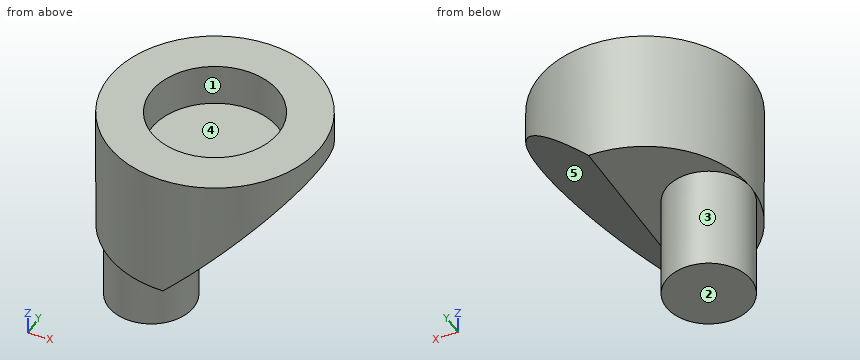
```python
from build123d import *

# Parameters (mm, degrees)
F0_R          = 2.5
F1_DEPTH      = 3
F3_DEPTH      = 25
F3_DEPTH_BACK = 25
F4_R          = 1
F5_DEPTH      = 2.5
F6_R          = 1.5
F7_DEPTH      = 1


with BuildPart() as f1:
    # F0 (on Top) → F1 (new body)
    with BuildSketch(Plane.XY):
        Circle(F0_R)
    extrude(amount=F1_DEPTH)

    # F2 (on Front) → F3 (cut, two sides)
    with BuildSketch(Plane.XZ) as f3_sk:
        Polygon((6.7282968301, 6.6747666272), (-4.7879227272, -4.8414529301), (6.7282968301, -4.8414529301), align=None)
    extrude(amount=-F3_DEPTH, mode=Mode.SUBTRACT)
    extrude(f3_sk.sketch, amount=F3_DEPTH_BACK, mode=Mode.SUBTRACT)

    # F4 (on face) → F5 (join)
    with BuildSketch(Plane(origin=(0, 0, 0), x_dir=(1, 0, 0), z_dir=(0, 0, -1))):
        with Locations((-1.5, 0)):
            Circle(F4_R)
    extrude(amount=F5_DEPTH)

    # F6 (on face) → F7 (cut)
    with BuildSketch(Plane.XY.offset(3)):
        Circle(F6_R)
    extrude(amount=-F7_DEPTH, mode=Mode.SUBTRACT)


solid = f1.part
```
Geometry: final body of the model. Coordinates: model frame, mm. Face numbers are marked on the shaded views. A direction names the side the tool comes from. Give positions to 0.01 mm unless a question says otherwise; leave off trailing zeros. Loops run counter-clockwise (first coordinate to the right, second up) from the corner with the lowest first, then second, coordinate; pieces in that order, holes last. Notation, with made-up numbers: (8, 54.25) -> (35, 54.25) arc R21 ccw to (35, 77.25) -> close; hole circle Ø2 at (23.25, 17.25). An arc over 180 degrees is marked (long way). Use CSV: the item, a comma, the result in double quotes.
(1) Cut plane B-B (x = -0.8). Output: boundary loops of the cut face in (y, z).
From the geometry:
outline,"(-2.37, 0) -> (-0.71, 0) -> (-0.71, -2.5) -> (0.71, -2.5) -> (0.71, 0) -> (2.37, 0) -> (2.37, 3) -> (1.27, 3) -> (1.27, 2) -> (-1.27, 2) -> (-1.27, 3) -> (-2.37, 3) -> close"
(2) Cut plane D-D (y = -1.15). Output: boundary loops of the cut face in (x, z).
From the geometry:
outline,"(-2.22, 0) -> (0.05, 0) -> (2.22, 2.17) -> (2.22, 3) -> (0.96, 3) -> (0.96, 2) -> (-0.96, 2) -> (-0.96, 3) -> (-2.22, 3) -> close"
(3) First-contact query: P1, Ø1.5, axis at y = 1, z = -1.5, coming from the +X side. Flat tip, straight axial feed; report the tip coordinate or a pass-through.
From the geometry:
P1,"x = -0.53"
(4) Pull-direction query (Y, two-part tool) for the marked faces 3, 4 and 5; classes: released by +Y, released by -Y, zero draft, split by the parting line, or undercut.
From the geometry:
face 3,"split by the parting line"
face 4,"undercut"
face 5,"zero draft"
(5) Cut plane C-C (z = 2.6). Output: boundary loops of the cut face in (x, y), plus the area to 3 significant figures.
From the geometry:
outline,"circle Ø5 at (0, 0); hole circle Ø3 at (0, 0)"
area,"12.6 mm^2"
(6) Access query for the marked faces 1 and 2. Directions: +Z, -Z, +X, -X, +Y, -Y. A direction counts if a zero-diameter tool reaches every point of the face in a straight line with its end or side. Return the directions, or none.
From the geometry:
face 1,"+Z"
face 2,"-Z, +X, -X, +Y, -Y"
(7) Ray query, line 1 along Y through (x, z) = (0, 2.55); line 2 along Z through (x, y) = (-0.85, -1.6); line 3 along X through (y, z) = (2, 1.5). Return the intervals inside material, ascending. Write a range as [from, to].
From the geometry:
line 1,"[-2.5, -1.5], [1.5, 2.5]"
line 2,"[0, 3]"
line 3,"[-1.5, 1.5]"
